Design review of the part built by this model. Coordinates are the model's own, in mm. Round coordinates to 2 decimals unless told otherwise and drop trailing zeros. Write each loop counter-clockwise with the first axis right and the second up, starting at its lowest first coordinate (ties: lowest second). Pieces come first, ordered by that corner, then holes. Notation, with made-up numbers: (-11.5, 27) - (-7.5, 27) arc R31 ccw to (-7.5, 63) - close; hole circle Ø8 at (46, 16). An arc over 180 degrees is marked (long way). Use one line per item in the form item = value.
Autodesk Inventor part; units mm, degrees
ref_plane "YZ Plane" through (0, 0, 0) normal (1, 0, 0) x (0, 1, 0)
ref_plane "XZ Plane" through (0, 0, 0) normal (0, 1, 0) x (-1, 0, 0)
ref_plane "XY Plane" through (0, 0, 0) normal (0, 0, 1) x (1, 0, 0)
sketch "Sketch1" plane through (0, 0, 0) normal (0, 1, 0) x (-1, 0, 0)
  line L0 (-32.5, -32.5) -> (32.5, -32.5)
  line L1 (32.5, -32.5) -> (32.5, 32.5)
  line L2 (32.5, 32.5) -> (-32.5, 32.5)
  line L3 (-32.5, 32.5) -> (-32.5, -32.5)
  line L4 (-32.5, -32.5) -> (32.5, 32.5) construction
  line L5 (32.5, -32.5) -> (-32.5, 32.5) construction
  line L6 (-21.5, -20) -> (21.5, -20) construction
  line L7 (21.5, -20) -> (21.5, 20) construction
  line L8 (21.5, 20) -> (-21.5, 20) construction
  line L9 (-21.5, 20) -> (-21.5, -20) construction
  line L10 (-21.5, -20) -> (21.5, 20) construction
  line L11 (21.5, -20) -> (-21.5, 20) construction
  circle A0 centre (21.5, 20) radius 2.5
  point P0 (0, 0)
  dimension "d0" = 65
  dimension "d1" = 65
  dimension "d5" = 43
  dimension "d6" = 40
  dimension "d7" = 5
extrude "Extrusion1" add sketch "Sketch1" along normal blind 3 contours L3 L2 L1 L0 | A0
fillet "Fillet1" radius 2 4 edges at (32.5, 1.5, 32.5) (32.5, 1.5, -32.5) (-32.5, 1.5, 32.5) (-32.5, 1.5, -32.5)
extrude "Extrusion2" cut sketch "Sketch1" along normal blind 3 contours A0
pattern_linear "Rectangular Pattern1" count 2 spacing 40 along (0, 0, -1) count 2 spacing 43 along (1, 0, 0) of "Extrusion2"
properties part number "wheel_plate"
Q1. We need section A-A on z = -20. Write out the cut boundary in (x, y), then the cut area to 3 significant figures.
Calculated:
outline = (-32.5, 0) - (-24, 0) - (-24, 3) - (-32.5, 3) - close; (-19, 0) - (19, 0) - (19, 3) - (-19, 3) - close; (24, 0) - (32.5, 0) - (32.5, 3) - (24, 3) - close
area = 165 mm2
Q2. Draft analysis for pull direction Z (two halves, no side actions). For faces 1 (the flat face through (0, 1, -32.5)), 2 (the flat face through (0, 3, 0)), 3 (the cylindrical face through (-20, 1, -22)), state which applies: released by +Z, released by -Z, zero draft, split by the parting line, or undercut.
Calculated:
face_1 = released by -Z
face_2 = zero draft
face_3 = undercut
Q3. We need section C-C on y = 2.35. Write out the cut boundary in (x, z), then the cut area to 3 significant figures.
Calculated:
outline = (-32.5, -30.5) arc R2 ccw to (-30.5, -32.5) - (30.5, -32.5) arc R2 ccw to (32.5, -30.5) - (32.5, 30.5) arc R2 ccw to (30.5, 32.5) - (-30.5, 32.5) arc R2 ccw to (-32.5, 30.5) - close; hole circle Ø5 at (-21.5, -20); hole circle Ø5 at (-21.5, 20); hole circle Ø5 at (21.5, -20); hole circle Ø5 at (21.5, 20)
area = 4,140 mm2
Q4. To check wall thickness, follow line 1 along Z through (x, y) = (-21.5, 1.8). State the ranges of the line that lie inside material, in increasing order. Write a range as from..to.
Calculated:
line_1 = -32.5..-22.5, -17.5..17.5, 22.5..32.5
Q5. For P1, Ø3, axis at x = 21.5, z = 20, coming from the +Y side, flat-tipped, find the tip position at first contact; note if it passes through.
Calculated:
P1 = through
Q6. We need section B-B on x = 21.5. Write out the cut boundary in (y, z), then the cut area to 3 significant figures.
Calculated:
outline = (0, -32.5) - (3, -32.5) - (3, -22.5) - (0, -22.5) - close; (0, -17.5) - (3, -17.5) - (3, 17.5) - (0, 17.5) - close; (0, 22.5) - (3, 22.5) - (3, 32.5) - (0, 32.5) - close
area = 165 mm2
